For this review, use the dimensioned drawing (mm, ordinates from the lowest corner) and the shaded views. Coordinates: 2 decimals unless noted, no trailing zeros. Order: outer loops, then holes, each group sorted by start corner. A loop starts at its lowest first (then second) coordinate and runs counter-clockwise, first axis right, second up. Notation, with made-up numbers: (-38.5, -38) -> (13.5, -38) arc R24 cw to (13.5, -25) -> close; hole circle Ø4 at (61, 61.25). An arc over 180 degrees is marked (long way). Use one line per item in the form item = value. Start each with the question number.
(1) Take a section at A-A (y = 7.25). State the section outline as (x, z) points, then the cut area to 3 significant figures.
(2) Wall thickness on line 1 along Y through (x, z) = (53.5, 3.1); line 2 along X through (y, z) = (16.25, 3.3): over which ranges is each line inside the solid? List them lowest first.
(3) Insertion check: pin 1 Ø2.5 at (x, z) = (54.5, 5) entering from +Y; pin 2 Ø0.9 at (y, z) = (8.5, 5) entering from -X; pin 3 Ø3.5 at (x, y) = (55, 9.5) entering from +Z. Each pin has a flat end and moves straight along its axis. Give the tip position at first contact, or say it passes through.
(4) Take a section at B-B (z = 5.1). State the section outline as (x, y) points.
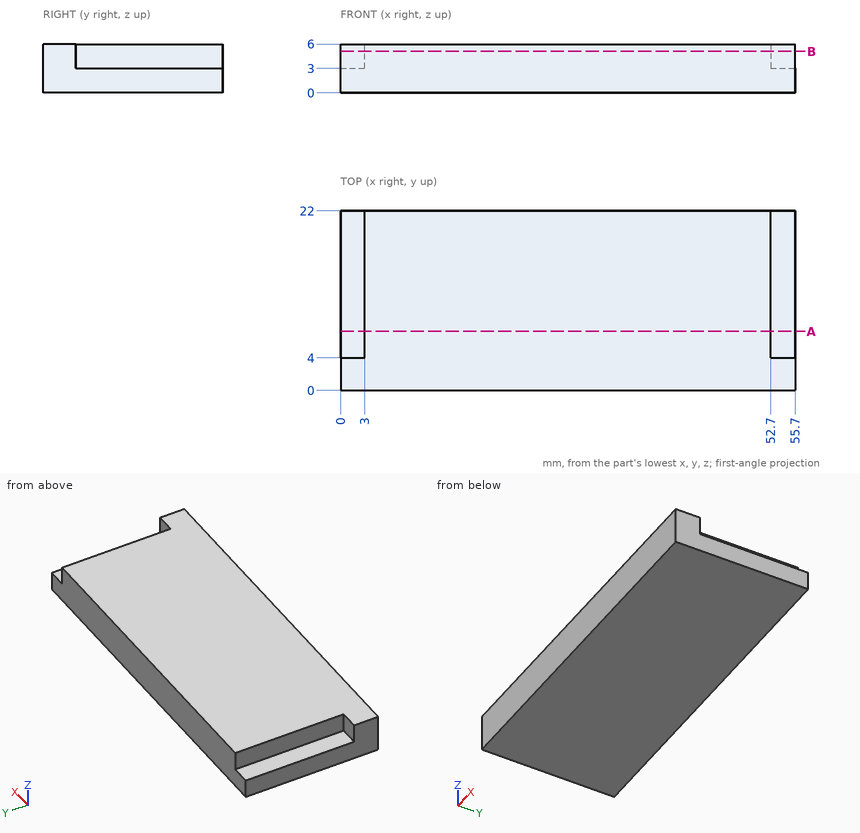
Findings:
q1.outline = (0, 0) -> (55.7, 0) -> (55.7, 3) -> (52.7, 3) -> (52.7, 6) -> (3, 6) -> (3, 3) -> (0, 3) -> close
q1.area = 316 mm²
q2.line_1 = 0 to 4
q2.line_2 = 3 to 52.7
q3.pin_1 = 4
q3.pin_2 = 3
q3.pin_3 = 3
q4.outline = (0, 0) -> (55.7, 0) -> (55.7, 4) -> (52.7, 4) -> (52.7, 22) -> (3, 22) -> (3, 4) -> (0, 4) -> close
